The model under review builds one solid part; all positions refer to its coordinate system, in mm. A direction names the side the tool comes from. Round coordinates to 2 decimals unless told otherwise and drop trailing zeros. Order: outer loops, then holes, each group sorted by start corner. A loop starts at its lowest first (then second) coordinate and runs counter-clockwise, first axis right, second up. Notation, with made-up numbers: M 77.25,68.5 L 105.25,68.5 A19 cw 105.25,94.5 Z; hole C 18,41 d7. An arc over 180 degrees is marked long. Answer as a JSON object with one key per item and string values. Group by question number.
1) Consider section D-D, the plane y = -15.5. Write out the cut boundary in (x, z) (1 decimal), then the cut area to 3 significant figures.
2) For faces 1 (the flat face through (0, -18, 3.175)), 2 (the flat face through (12, 0, 0)), list the 3-axis set-ups (+Z, -Z, +X, -X, +Y, -Y) from which the entire face can be reached by the end or side of a thin tool; tool diameter is ignored.
3) Consider section B-B, the plane x = -8.5. Write out the cut boundary in (y, z) (1 decimal).
4) Consider section A-A, the plane y = 0. Write out the cut boundary in (x, z) (1 decimal), then the cut area to 3 significant figures.
5) The part is to be moulded in two halves that separate along X. For faces 3 (the flat face through (-0.2, -11.4, 7.938)), 4 (the cylindrical face through (-19.89, 18.24, 1.57)), 5 (the cylindrical face through (-10.6, 3.34, 3.91)), say which applies: +X half, -X half, draft (parallel to the pull), parting line (faces both ways), or undercut.
6) Insertion check: pin 1 Ø1.5 at (y, z) = (-17, 2) entering from +X; pin 2 Ø3 at (x, y) = (-11.5, 15.5) entering from +Z (3 decimals); pin 3 Ø1.5 at (x, z) = (-10, 2) entering from +Y. Each pin has a flat end and moves straight along its axis. Give the tip position at first contact, or say it passes through.
7) Consider section C-C, the plane z = 4.5. Write out the cut boundary in (x, y) (1 decimal), then the cut area to 3 significant figures.
8) To check wall thickness, follow line 1 (Y direction, x = 0, z = 3.5); line 2 (Y direction, x = 0, z = 2.25); line 3 (Z direction, x = -21, y = -16) (3 decimals). State the ranges of each line that lie inside material, in increasing order.
```python
from build123d import *

# Parameters (mm, degrees)
F0_R     = 26.9875
F1_DEPTH = 3.175
F2_R     = 17.4625
F3_DEPTH = 4.7625
F5_D     = 22.225


with BuildPart() as f1:
    # F0 (on Top) → F1 (new body)
    with BuildSketch(Plane.XY):
        Circle(F0_R)
    extrude(amount=F1_DEPTH)

    # F2 (on face) → F3 (join)
    with BuildSketch(Plane.XY.offset(3.175)):
        Circle(F2_R)
    extrude(amount=F3_DEPTH)

    # F5 (through all)
    with Locations(Plane.XY.offset(7.9375)):
        with Locations((0, 0)):
            Hole(F5_D / 2)


solid = f1.part
```
Results list:
{
 "1": {"outline": "M -22.1,0 L 22.1,0 L 22.1,3.2 L 8,3.2 L 8,7.9 L -8,7.9 L -8,3.2 L -22.1,3.2 Z", "area": "217 mm^2"},
 "2": {"face 1": "+Z", "face 2": "-Z, +X, -X, +Y, -Y"},
 "3": {"outline": "M -25.6,0 L -7.2,0 L -7.2,7.9 L -15.3,7.9 L -15.3,3.2 L -25.6,3.2 Z; M 7.2,0 L 25.6,0 L 25.6,3.2 L 15.3,3.2 L 15.3,7.9 L 7.2,7.9 Z"},
 "4": {"outline": "M -27,0 L -11.1,0 L -11.1,7.9 L -17.5,7.9 L -17.5,3.2 L -27,3.2 Z; M 11.1,0 L 27,0 L 27,3.2 L 17.5,3.2 L 17.5,7.9 L 11.1,7.9 Z", "area": "161 mm^2"},
 "5": {"face 3": "draft", "face 4": "parting line", "face 5": "undercut"},
 "6": {"pin 1": "x = 21.55", "pin 2": "z = 3.175", "pin 3": "y = 25.35"},
 "7": {"outline": "C 0,0 d34.9; hole C 0,0 d22.2", "area": "570 mm^2"},
 "8": {"line 1": "-17.46 to -11.11, 11.11 to 17.46", "line 2": "-26.99 to -11.11, 11.11 to 26.99", "line 3": "0 to 3.175"}
}
